from build123d import *

# Parameters (mm, degrees)
BOSS_EXTRU_1_DEPTH      = 17
ESQUISSE2_R             = 1.3
ENL_V_MAT_EXTRU_1_DEPTH = 17
ESQUISSE3_R             = 9
ESQUISSE3_R_2           = 1.3
BOSS_EXTRU_2_DEPTH      = 10
ESQUISSE4_W             = 0.84262724
ESQUISSE4_H             = 4.751474998
ENL_V_MAT_EXTRU_2_DEPTH = 12
ESQUISSE5_R             = 1.3
ENL_V_MAT_EXTRU_3_DEPTH = 27
ESQUISSE6_R             = 2.1
ENL_V_MAT_EXTRU_4_DEPTH = 10


with BuildPart() as part:
    # Esquisse1 → Boss.-Extru.1 (new body)
    with BuildSketch(Plane.XY):
        Polygon((6, 3.464101615), (0, 6.92820323), (-6, 3.464101615), (-6, -3.464101615), (0, -6.92820323), (6, -3.464101615), align=None)
    extrude(amount=BOSS_EXTRU_1_DEPTH)

    # Esquisse2 → Enlèv. mat.-Extru.1 (cut)
    with BuildSketch(Plane.XY.offset(17)):
        Circle(ESQUISSE2_R)
    extrude(amount=-ENL_V_MAT_EXTRU_1_DEPTH, mode=Mode.SUBTRACT)

    # Esquisse3 → Boss.-Extru.2 (add)
    with BuildSketch(Plane.XY.offset(17)):
        Circle(ESQUISSE3_R)
        Circle(ESQUISSE3_R_2, mode=Mode.SUBTRACT)
    extrude(amount=-BOSS_EXTRU_2_DEPTH)

    # Esquisse4 → Enlèv. mat.-Extru.2 (cut)
    with BuildSketch(Plane.XY.offset(17)):
        with Locations((9, 0)):
            Rectangle(ESQUISSE4_W, ESQUISSE4_H)
    extrude(amount=-ENL_V_MAT_EXTRU_2_DEPTH, mode=Mode.SUBTRACT)

    # Esquisse5 → Enlèv. mat.-Extru.3 (cut)
    with BuildSketch(Plane(origin=(8.57868638, 0, 0), x_dir=(0, 0, -1), z_dir=(1, 0, 0))):
        with Locations((-12, 0)):
            Circle(ESQUISSE5_R)
    extrude(amount=-ENL_V_MAT_EXTRU_3_DEPTH, mode=Mode.SUBTRACT)

    # Esquisse6 → Enlèv. mat.-Extru.4 (cut)
    with BuildSketch(Plane.XY.offset(17)):
        Circle(ESQUISSE6_R)
    extrude(amount=-ENL_V_MAT_EXTRU_4_DEPTH, mode=Mode.SUBTRACT)


solid = part.part
Geometry: final body of the model. Coordinates: model frame, mm. A direction names the side the tool comes from. Coordinates: 2 decimals unless noted, no trailing zeros. Write each loop counter-clockwise with the first axis right and the second up, starting at its lowest first coordinate (ties: lowest second). Pieces come first, ordered by that corner, then holes. Notation, with made-up numbers: (30.25, 53.25) - (56.25, 53.25) arc R19 ccw to (56.25, 65.25) - close; hole circle Ø1 at (21.25, 11). An arc over 180 degrees is marked (long way). Return JSON: item names as keys, results as strings.
Item 1: Line query: L1, parallel to Z at x = -4.75, y = 0; L2, parallel to X at y = 1.25, z = 14.75; L3, parallel to Z at x = -7.5, y = 0. Output: solid intervals per line, ascending.
Completed:
{"L1": "z = 0 to 10.7, 13.3 to 17", "L2": "x = -8.91 to -1.69, 1.69 to 8.58", "L3": "z = 7 to 10.7, 13.3 to 17"}
Item 2: Section query D-D (x = 3). Output: boundary loops of the cut face in (y, z).
Completed:
{"outline": "(-8.49, 7) - (-5.2, 7) - (-5.2, 0) - (5.2, 0) - (5.2, 7) - (8.49, 7) - (8.49, 17) - (-8.49, 17) - close; hole circle Ø2.6 at (0, 12)"}
Item 3: Section query C-C (z = 2.25). Output: boundary loops of the cut face in (x, y), and give its area (3 significant figures).
Completed:
{"outline": "(-6, -3.46) - (0, -6.93) - (6, -3.46) - (6, 3.46) - (0, 6.93) - (-6, 3.46) - close; hole circle Ø2.6 at (0, 0)", "area": "119 mm2"}
Item 4: Pin query (flat end, axial travel): pin 1 Ø2 at (x, z) = (-5, 10) entering from -Y; pin 2 Ø1 at (x, z) = (-2.5, 2.5) entering from -Y; pin 3 Ø3.5 at (x, y) = (0, 0) entering from +Z. Return the tip coordinate at first contact, or that it passes through.
Completed:
{"pin 1": "stops at y = -8.06", "pin 2": "stops at y = -5.77", "pin 3": "stops at z = 7"}
Item 5: Section query A-A (y = 0). Output: boundary loops of the cut face in (x, z), and give its area (3 significant figures).
Completed:
{"outline": "(-9, 7) - (-6, 7) - (-6, 0) - (-1.3, 0) - (-1.3, 7) - (-2.1, 7) - (-2.1, 10.7) - (-9, 10.7) - close; (-9, 13.3) - (-2.1, 13.3) - (-2.1, 17) - (-9, 17) - close; (1.3, 0) - (6, 0) - (6, 7) - (8.58, 7) - (8.58, 10.7) - (2.1, 10.7) - (2.1, 7) - (1.3, 7) - close; (2.1, 13.3) - (8.58, 13.3) - (8.58, 17) - (2.1, 17) - close", "area": "165 mm2"}
Item 6: Pull-direction query (Y, two-part tool) for faces 1 (the face through (3.042, 5.172, 3.451)), 2 (the face through (-0.17, 1.29, 3.55)), 3 (the face through (-6, 0, 3)); classes: +Y half, -Y half, draft (parallel to the pull), parting line (faces both ways), or undercut.
Completed:
{"face 1": "+Y half", "face 2": "undercut", "face 3": "draft"}
Item 7: Section query B-B (z = 12). Output: boundary loops of the cut face in (x, y).
Completed:
{"outline": "(-8.91, -1.3) arc R9 ccw to (8.68, -2.38) - (8.58, -2.38) - (8.58, -1.3) - (1.65, -1.3) arc R2.1 cw to (-1.65, -1.3) - close; (-8.91, 1.3) - (-1.65, 1.3) arc R2.1 cw to (1.65, 1.3) - (8.58, 1.3) - (8.58, 2.38) - (8.68, 2.38) arc R9 ccw to start"}
Item 8: Reachability of faces 4 (the face through (1.13, 1.77, 12.07)), 5 (the face through (-6.2, 0.1, 7)), 6 (the face through (2.96, -5.22, 3.45)), 7 (the face through (6, 0, 3)), 8 (the face through (-2.96, 5.22, 3.45)) from +Z, -Z, +X, -X, +Y, -Y: full face, straight path, thin tool, end or side. Return the list, or none.
Completed:
{"face 4": "+Z", "face 5": "-Z", "face 6": "-Z, +X, -Y", "face 7": "-Z, +X, +Y, -Y", "face 8": "-Z, -X, +Y"}
